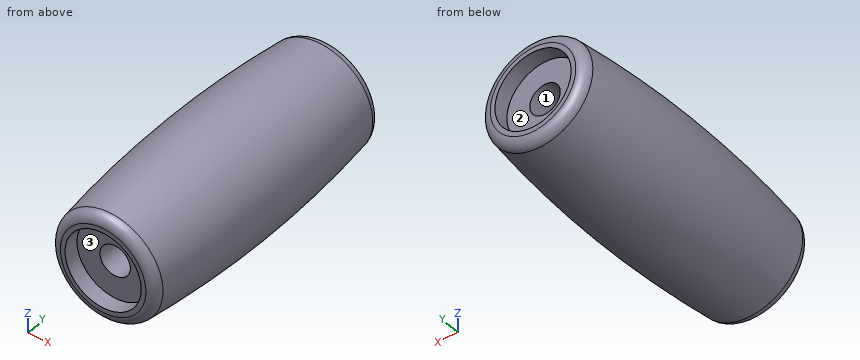
from build123d import *

# Parameters (mm, degrees)
SKETCH2_R          = 3.75
CUT_EXTRUDE1_DEPTH = 1.5
SKETCH3_R          = 3.75
CUT_EXTRUDE2_DEPTH = 1.5
SKETCH4_R          = 1.5
CUT_EXTRUDE3_DEPTH = 27.5


with BuildPart() as part:
    # Sketch1 → Revolve1 (revolve)
    with BuildSketch(Plane.XY):
        with BuildLine():
            Line((0, 0), (-4.209254706, 0))
            ThreePointArc((-4.209254706, 0), (-4.872125478, 0.251266175), (-5.201882242, 0.87879532))
            ThreePointArc((-5.201882242, 0.87879532), (-6, 14), (-5.201882242, 27.12120468))
            ThreePointArc((-5.201882242, 27.12120468), (-4.872125478, 27.748733825), (-4.209254706, 28))
            Line((-4.209254706, 28), (0, 28))
            Line((0, 28), (0, 0))
        make_face()
    revolve(axis=Axis((0, 0, 0), (0, 1, 0)))

    # Sketch2 → Cut-Extrude1 (cut)
    with BuildSketch(Plane(origin=(0, 28, 0), x_dir=(1, 0, 0), z_dir=(0, 1, 0))):
        Circle(SKETCH2_R)
    extrude(amount=-CUT_EXTRUDE1_DEPTH, mode=Mode.SUBTRACT)

    # Sketch3 → Cut-Extrude2 (cut)
    with BuildSketch(Plane.XZ):
        Circle(SKETCH3_R)
    extrude(amount=-CUT_EXTRUDE2_DEPTH, mode=Mode.SUBTRACT)

    # Sketch4 → Cut-Extrude3 (cut, through all)
    with BuildSketch(Plane(origin=(0, 1.5, 0), x_dir=(-1, 0, 0), z_dir=(0, -1, 0))):
        Circle(SKETCH4_R)
    extrude(amount=-CUT_EXTRUDE3_DEPTH, mode=Mode.SUBTRACT)


solid = part.part
Verification items for the finished model (mm, model axes). Face numbers are marked on the shaded views. A direction names the side the tool comes from. Round coordinates to 2 decimals unless told otherwise and drop trailing zeros. Use a Markdown table: item, result. Add a question column.
1. Access from +Z, -Z, +X, -X, +Y, -Y to the whole of each face (thin tool, end or side, straight path). Record for the marked faces 1, 2 and 3.
2. Thickness scan on probe 1 along Y at (x, z) = (-2.75, 3.25); probe 2 along X at (y, z) = (14.25, 0.5); probe 3 along X at (y, z) = (7.25, 0). Record the ranges inside material, lowest first. Write a range as [from, to].
3. Gauge pin test, flat ends, axial feed: pin 1 (2 mm diameter, centred on x = 0.5, z = -1, fed in from -Y); pin 2 (4 mm diameter, centred on x = -4.5, y = 20, fed in from -Z); pin 3 (1 mm diameter, centred on x = 4.5, y = 12.5, fed in from -Z). Record the tip position at first contact, or that the pin passes through.
Checks:
| question | item | result |
|---|---|---|
| 1 | face 1 | +Y, -Y |
| 1 | face 2 | +Y |
| 1 | face 3 | -Y |
| 2 | probe 1 | y = [0, 28] |
| 2 | probe 2 | x = [-5.98, -1.41], [1.41, 5.98] |
| 2 | probe 3 | x = [-5.79, -1.5], [1.5, 5.79] |
| 3 | pin 1 | stops at y = 1.5 |
| 3 | pin 2 | stops at z = -5.28 |
| 3 | pin 3 | stops at z = -4.46 |
